Input: dimensioned drawing with shaded views. Units: mm. Origin: part minimum x, y, z. A direction names the side the tool comes from. Coordinates: 2 decimals unless noted, no trailing zeros. Loops run counter-clockwise (first coordinate to the right, second up) from the corner with the lowest first, then second, coordinate; pieces in that order, holes last.
(1) Contact query for a flat-ended pin moving along its axis: P1, Ø6, axis at x = 62, y = 28, coming from the +Z side. Output: stop coordinate, or through.
(2) Line query: L1, parallel to Y at x = 100, z = 1.55; L2, parallel to X at y = 25.5, z = 4.75; L3, parallel to X at y = 28.5, z = 4. Output: solid intervals per line, ascending.
(3) Section D-D, the plane x = 78. Return loops of the section in (y, z).
(4) Section B-B, the plane x = 100. Return loops of the section in (y, z).
(5) Section A-A, the plane y = 39. Return loops of the section in (x, z), then the cut area to 3 significant figures.
(6) Set-up query: the marked faces 1, 2, 3, 4 and 5. Return all of +Z, -Z, +X, -X, +Y, -Y with unobstructed straight access to the full face (end or side cutting, diameter ignored); none if empty.
(7) Section C-C, the plane x = 20. Return loops of the section in (y, z), then the cut area to 3 significant figures.
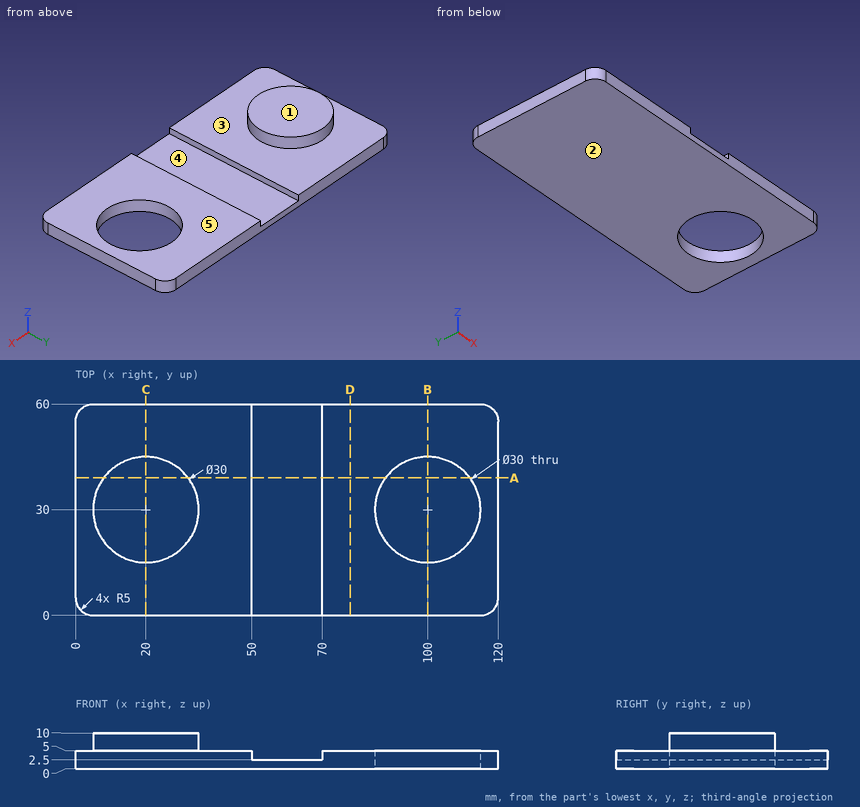
Report:
1. P1: stops at z = 2.5
2. L1: y = 0 to 15, 45 to 60
2. L2: x = 0 to 50, 70 to 85.69, 114.31 to 120
2. L3: x = 0 to 50, 70 to 85.08, 114.92 to 120
3. outline: (0, 0) - (60, 0) - (60, 5) - (0, 5) - close
4. outline: (0, 0) - (15, 0) - (15, 5) - (0, 5) - close; (45, 0) - (60, 0) - (60, 5) - (45, 5) - close
5. outline: (0, 0) - (88, 0) - (88, 5) - (70, 5) - (70, 2.5) - (50, 2.5) - (50, 5) - (32, 5) - (32, 10) - (8, 10) - (8, 5) - (0, 5) - close; (112, 0) - (120, 0) - (120, 5) - (112, 5) - close
5. area: 550 mm2
6. face 1: +Z, +X, -X, +Y, -Y
6. face 2: -Z, +X, -X, +Y, -Y
6. face 3: +Z
6. face 4: +Z, +Y, -Y
6. face 5: +Z, +X, +Y, -Y
7. outline: (0, 0) - (60, 0) - (60, 5) - (45, 5) - (45, 10) - (15, 10) - (15, 5) - (0, 5) - close
7. area: 450 mm2
